```python
from build123d import *

# Parameters (mm, degrees)
SKETCH_1_R               = 3
EXTRUDE_1_DEPTH          = 2.4
SKETCH_2_R               = 1.75
EXTRUDE_2_DEPTH          = 38
CHAMFER_1_SIZE           = 0.3355
SKETCH_3_W               = 1.2
SKETCH_3_H               = 1.2
CUT_EXTRUDE_1_DEPTH      = 38
CUT_EXTRUDE_1_DEPTH_BACK = 38


with BuildPart() as part:
    # Sketch 1 → Extrude 1 (new body)
    with BuildSketch(Plane.XY):
        Circle(SKETCH_1_R)
    extrude(amount=EXTRUDE_1_DEPTH)

    # Sketch 2 → Extrude 2 (add)
    with BuildSketch(Plane(origin=(0, 0, 0), x_dir=(-1, 0, 0), z_dir=(0, 0, -1))):
        Circle(SKETCH_2_R)
    extrude(amount=EXTRUDE_2_DEPTH)

    # Chamfer 1
    chamfer_1_edges = [part.edges().sort_by_distance(p)[0] for p in [
        (1.75, 0, -38),
    ]]
    chamfer(chamfer_1_edges, length=CHAMFER_1_SIZE)

    # Sketch 3 → Cut-Extrude 1 (cut, two sides)
    with BuildSketch(Plane(origin=(0, 0, 0), x_dir=(1, 0, 0), z_dir=(0, 1, 0))) as cut_extrude_1_sk:
        with Locations((0, -2.4)):
            Rectangle(SKETCH_3_W, SKETCH_3_H)
    extrude(amount=CUT_EXTRUDE_1_DEPTH, mode=Mode.SUBTRACT)
    extrude(cut_extrude_1_sk.sketch, amount=-CUT_EXTRUDE_1_DEPTH_BACK, mode=Mode.SUBTRACT)


solid = part.part
```
Geometry check sheet. Reference: the model listing, model coordinates, mm. A direction names the side the tool comes from. Give positions to 0.01 mm unless a question says otherwise; leave off trailing zeros. Loops run counter-clockwise (first coordinate to the right, second up) from the corner with the lowest first, then second, coordinate; pieces in that order, holes last. Notation, with made-up numbers: M 64,63.5 L 118,63.5 A17 ccw 118,92.5 Z; hole C -8,2 d4. An arc over 180 degrees is marked long. Write item = value, one per line. Start each with the question number.
1. Section check B-B, the plane x = 0. Enter the section's corners in (y, z), plus the area to 3 significant figures.
2. Section check C-C, the plane z = 0.5. Enter the section's corners in (x, y), plus the area to 3 significant figures.
3. Draft check along X on faces 3 (the face through (-1.617, -0.67, -18.569)), 4 (the face through (0, 0, 1.8)), 5 (the face through (2, 0, 2.4)). Enter one of: +X half, -X half, draft (parallel to the pull), parting line (faces both ways), or undercut.
4. Thickness scan on probe 1 along Z at (x, y) = (-0.05, 0.2); probe 2 along Z at (x, y) = (-1.4, 1.8); probe 3 along X at (y, z) = (0.1, -22). Record the ranges inside material, lowest first.
5. Tool access check on faces 1 (the face through (0, -2, 0)), 2 (the face through (-2, 0, 2.4)). Record the directions out of +Z, -Z, +X, -X, +Y, -Y that give a thin tool (end or side, any length) a straight path to the whole face; none if there is none.
6. Section check D-D, the plane z = -28. Enter the section's corners in (x, y), plus the area to 3 significant figures.
7. Section check A-A, the plane y = 0. Enter the section's corners in (x, z).
8. Go/stop test with flat-tipped pins: P1, Ø0.7, axis at y = -0.5, z = 2, coming from the +X side; P2, Ø0.7, axis at y = 1.5, z = 2, coming from the -X side; P3, Ø0.6, axis at x = 0, y = -1.5, coming from the +Z side. Record where each tip stops, or that it passes through.
Values follow:
q1.outline = M -3,0 L -1.75,0 L -1.75,-37.66 L -1.41,-38 L 1.41,-38 L 1.75,-37.66 L 1.75,0 L 3,0 L 3,1.8 L -3,1.8 Z
q1.area = 144 mm^2
q2.outline = C 0,0 d6
q2.area = 28.3 mm^2
q3.face_3 = parting line
q3.face_4 = undercut
q3.face_5 = draft
q4.probe_1 = -38 to 1.8
q4.probe_2 = 0 to 2.4
q4.probe_3 = -1.75 to 1.75
q5.face_1 = -Z
q5.face_2 = +Z, +X, -X, +Y, -Y
q6.outline = C 0,0 d3.5
q6.area = 9.62 mm^2
q7.outline = M -3,0 L -1.75,0 L -1.75,-37.66 L -1.41,-38 L 1.41,-38 L 1.75,-37.66 L 1.75,0 L 3,0 L 3,2.4 L 0.6,2.4 L 0.6,1.8 L -0.6,1.8 L -0.6,2.4 L -3,2.4 Z
q8.P1 = 3
q8.P2 = -2.77
q8.P3 = 1.8
